Geometry: see drawing. Coordinates: mm, zero at the bounding-box minimum. A direction names the side the tool comes from. Give positions to 0.01 mm unless a question says otherwise; leave off trailing zeros. Order: outer loops, then holes, each group sorted by start corner. A loop starts at its lowest first (then second) coordinate and runs counter-clockwise, first axis right, second up. Notation, with made-up numbers: (-8, 50.5) - (4, 50.5) arc R31 ccw to (4, 86.5) - close; hole circle Ø11 at (49.5, 14). An arc over 180 degrees is marked (long way). Write item = value, one per line. Start each with the question number.
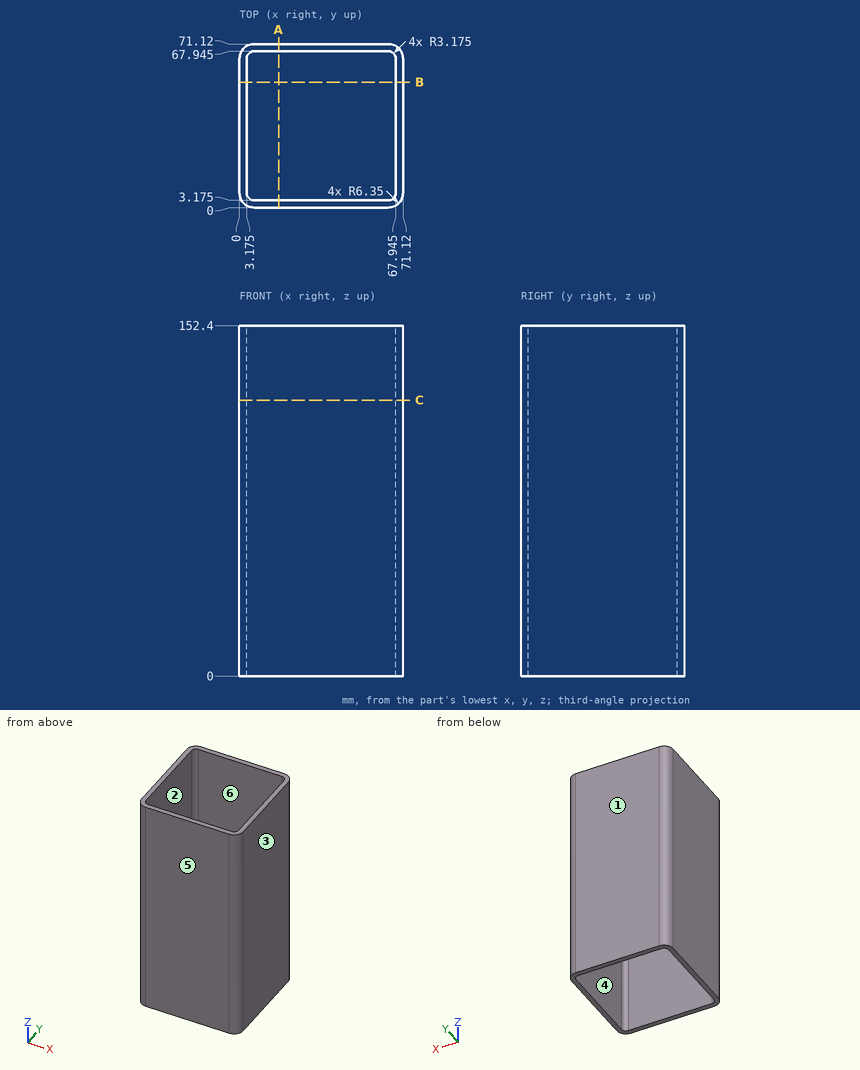
Q1. Set-up query: the marked faces 5 and 6. Return all of +Z, -Z, +X, -X, +Y, -Y with unobstructed straight access to the full face (end or side cutting, diameter ignored); none if empty.
Q2. Section C-C, the plane z = 120. Return the cut outline in (x, y) (3 decimals).
Q3. Pull-direction query (Y, two-part tool) for the marked faces 1, 2, 3 and 4; classes: +Y half, -Y half, draft (parallel to the pull), parting line (faces both ways), or undercut.
Q4. Section A-A, the plane x = 17. Return the cut outline in (y, z) (3 decimals), then the cut area to 3 significant figures.
Q5. Material intervals for line 1 along Y through (x, z) = (62.5, 126) (3 decimals), sorted ascending. Write a range as from..to.
The answers:
q1.face_5 = +Z, -Z, +X, -X, -Y
q1.face_6 = +Z, -Z
q2.outline = (0, 6.35) arc R6.35 ccw to (6.35, 0) - (64.77, 0) arc R6.35 ccw to (71.12, 6.35) - (71.12, 64.77) arc R6.35 ccw to (64.77, 71.12) - (6.35, 71.12) arc R6.35 ccw to (0, 64.77) - close; hole (3.175, 6.35) arc R3.175 ccw to (6.35, 3.175) - (64.77, 3.175) arc R3.175 ccw to (67.945, 6.35) - (67.945, 64.77) arc R3.175 ccw to (64.77, 67.945) - (6.35, 67.945) arc R3.175 ccw to (3.175, 64.77) - close
q3.face_1 = +Y half
q3.face_2 = undercut
q3.face_3 = draft
q3.face_4 = undercut
q4.outline = (0, 0) - (3.175, 0) - (3.175, 152.4) - (0, 152.4) - close; (67.945, 0) - (71.12, 0) - (71.12, 152.4) - (67.945, 152.4) - close
q4.area = 968 mm²
q5.line_1 = 0..3.175, 67.945..71.12
